```python
from build123d import *

# Parameters (mm, degrees)
SKETCH4_W                       = 152.4
SKETCH4_H                       = 101.6
BOSS_EXTRUDE3_DEPTH             = 6.35
SKETCH5_W                       = 101.6
SKETCH5_H                       = 101.6
BOSS_EXTRUDE4_DEPTH             = 95.25
SKETCH6_W                       = 76.2
SKETCH6_H                       = 76.2
CUT_EXTRUDE1_DEPTH              = 95.25
SKETCH7_R                       = 44.45
BOSS_EXTRUDE5_DEPTH             = 6.35
SKETCH8_R                       = 34.925
CUT_EXTRUDE3_DEPTH              = 171.861025398
CIRPATTERN1_COUNT               = 6
FILLET1_R                       = 3.81
F_4_40_TAPPED_HOLE1_D           = 2.2606
F_4_40_TAPPED_HOLE1_DEPTH       = 8.8646
F_4_40_TAPPED_HOLE1_CSINK_D     = 4.1148
F_4_40_TAPPED_HOLE1_CSINK_ANGLE = 90
F_4_40_TAPPED_HOLE1_TIP         = 0.679152758
SKETCH16_R                      = 19.05
BOSS_EXTRUDE6_DEPTH             = 2.54
CUT_EXTRUDE4_DEPTH              = 175.267880288
CUT_EXTRUDE4_DEPTH_BACK         = 175.267880288
SKETCH17_R                      = 12.7
CUT_EXTRUDE5_DEPTH              = 135.703841816
LPATTERN1_COUNT                 = 2
LPATTERN1_PITCH                 = 76.2


with BuildPart() as part:
    # Sketch4 → Boss-Extrude3 (new body)
    with BuildSketch(Plane(origin=(0, 0, 0), x_dir=(1, 0, 0), z_dir=(0, 1, 0))):
        Rectangle(SKETCH4_W, SKETCH4_H)
    extrude(amount=BOSS_EXTRUDE3_DEPTH)

    # Sketch5 → Boss-Extrude4 (add)
    with BuildSketch(Plane(origin=(0, 6.35, 0), x_dir=(1, 0, 0), z_dir=(0, 1, 0))):
        Rectangle(SKETCH5_W, SKETCH5_H)
    extrude(amount=BOSS_EXTRUDE4_DEPTH)

    # Sketch6 → Cut-Extrude1 (cut)
    with BuildSketch(Plane(origin=(0, 101.6, 0), x_dir=(1, 0, 0), z_dir=(0, 1, 0))):
        Rectangle(SKETCH6_W, SKETCH6_H)
    extrude(amount=-CUT_EXTRUDE1_DEPTH, mode=Mode.SUBTRACT)

    # Sketch7 → Boss-Extrude5 (add)
    with BuildSketch(Plane.XY.offset(50.8)):
        with Locations((0, 50.8)):
            Circle(SKETCH7_R)
    boss_extrude5 = extrude(amount=BOSS_EXTRUDE5_DEPTH)

    # Mirror2: Boss-Extrude5 across plane
    add(boss_extrude5.mirror(Plane.XY))

    # Sketch8 → Cut-Extrude3 (cut, through all)
    with BuildSketch(Plane.XY.offset(57.15)):
        with Locations((0, 50.8)):
            Circle(SKETCH8_R)
    extrude(amount=-CUT_EXTRUDE3_DEPTH, mode=Mode.SUBTRACT)

    # Sketch13 → 1/4-20 Tapped Hole2 (revolve, cut)
    with BuildSketch(Plane(origin=(39.6875, 50.8, 57.15), x_dir=(0, -1, 0), z_dir=(1, 0, 0))):
        Polygon((0, 0), (0, 20.583816902), (2.5527, 19.05), (2.5527, 1.2573), (3.81, 0), align=None)
    f_1_4_20_tapped_hole2 = revolve(axis=Axis((39.6875, 50.8, 63.5), (0, 0, -1)), mode=Mode.SUBTRACT)

    # CirPattern1: 1/4-20 Tapped Hole2 ×6 about axis
    cirpattern1_axis = Axis((0, 50.8, 0), (0, 0, 1))
    for i in range(1, CIRPATTERN1_COUNT):
        add(f_1_4_20_tapped_hole2.rotate(cirpattern1_axis, i * 360 / CIRPATTERN1_COUNT), mode=Mode.SUBTRACT)

    # Fillet1
    fillet1_edges = [part.edges().sort_by_distance(p)[0] for p in [
        (50.8, 53.975, 50.8),
        (50.8, 53.975, -50.8),
        (-50.8, 53.975, -50.8),
        (-50.8, 53.975, 50.8),
    ]]
    fillet(fillet1_edges, radius=FILLET1_R)

    # #4-40 Tapped Hole1
    with Locations(Plane(origin=(0, 101.6, 0), x_dir=(1, 0, 0), z_dir=(0, 1, 0))):
        with Locations((-46.99, 46.99), (46.99, 46.99), (46.99, -46.99), (-46.99, -46.99)):
            CounterSinkHole(F_4_40_TAPPED_HOLE1_D / 2, F_4_40_TAPPED_HOLE1_CSINK_D / 2, depth=F_4_40_TAPPED_HOLE1_DEPTH, counter_sink_angle=F_4_40_TAPPED_HOLE1_CSINK_ANGLE)
            with Locations((0, 0, -(F_4_40_TAPPED_HOLE1_DEPTH + F_4_40_TAPPED_HOLE1_TIP / 2))):  # 118° drill point
                Cone(0, F_4_40_TAPPED_HOLE1_D / 2, F_4_40_TAPPED_HOLE1_TIP, mode=Mode.SUBTRACT)

    # Sketch16 → Boss-Extrude6 (add)
    with BuildSketch(Plane(origin=(50.8, 0, 0), x_dir=(0, 0, -1), z_dir=(1, 0, 0))):
        with Locations(Location((0, 76.2, 0), (0, 0, 180))):
            Circle(SKETCH16_R)
    boss_extrude6 = extrude(amount=BOSS_EXTRUDE6_DEPTH)

    # Mirror4: Boss-Extrude6 across plane
    add(boss_extrude6.mirror(Plane(origin=(0, 0, 0), x_dir=(0, 0, 1), z_dir=(1, 0, 0))))

    # Sketch17 → Cut-Extrude4 (cut, two sides: drawn at the far end of the back side and taken through both)
    with BuildSketch(Plane(origin=(53.34, 0, 0), x_dir=(0, 0, -1), z_dir=(1, 0, 0)).offset(-CUT_EXTRUDE4_DEPTH_BACK)):
        with Locations(Location((0, 76.2, 0), (0, 0, 180))):
            Circle(SKETCH17_R)
    extrude(amount=CUT_EXTRUDE4_DEPTH + CUT_EXTRUDE4_DEPTH_BACK, mode=Mode.SUBTRACT)

    # Mirror5: 1/4-20 Tapped Hole2 across plane
    add(f_1_4_20_tapped_hole2.mirror(Plane.XY), mode=Mode.SUBTRACT)

    # Mirror5 copy 1 sketch → Mirror5 copy 1 (revolve, cut)
    with BuildSketch(Plane(origin=(19.84375, 85.170383213, -57.15), x_dir=(0.8660254037844386, -0.5000000000000001, 0), z_dir=(0.5000000000000001, 0.8660254037844386, 0))):
        Polygon((0, 0), (0, -20.583816902), (2.5527, -19.05), (2.5527, -1.2573), (3.81, 0), align=None)
    revolve(axis=Axis((19.84375, 85.170383213, -63.5), (0, 0, -1)), mode=Mode.SUBTRACT)

    # Mirror5 copy 2 sketch → Mirror5 copy 2 (revolve, cut)
    with BuildSketch(Plane(origin=(-19.84375, 85.170383213, -57.15), x_dir=(0.8660254037844387, 0.4999999999999998, 0), z_dir=(-0.4999999999999998, 0.8660254037844387, 0))):
        Polygon((0, 0), (0, -20.583816902), (2.5527, -19.05), (2.5527, -1.2573), (3.81, 0), align=None)
    revolve(axis=Axis((-19.84375, 85.170383213, -63.5), (0, 0, -1)), mode=Mode.SUBTRACT)

    # Mirror5 copy 3 sketch → Mirror5 copy 3 (revolve, cut)
    with BuildSketch(Plane(origin=(-39.6875, 50.8, -57.15), x_dir=(0, 1, 0), z_dir=(-1, 0, 0))):
        Polygon((0, 0), (0, -20.583816902), (2.5527, -19.05), (2.5527, -1.2573), (3.81, 0), align=None)
    revolve(axis=Axis((-39.6875, 50.8, -63.5), (0, 0, -1)), mode=Mode.SUBTRACT)

    # Mirror5 copy 4 sketch → Mirror5 copy 4 (revolve, cut)
    with BuildSketch(Plane(origin=(-19.84375, 16.429616787, -57.15), x_dir=(-0.8660254037844384, 0.5000000000000004, 0), z_dir=(-0.5000000000000004, -0.8660254037844384, 0))):
        Polygon((0, 0), (0, -20.583816902), (2.5527, -19.05), (2.5527, -1.2573), (3.81, 0), align=None)
    revolve(axis=Axis((-19.84375, 16.429616787, -63.5), (0, 0, -1)), mode=Mode.SUBTRACT)

    # Mirror5 copy 5 sketch → Mirror5 copy 5 (revolve, cut)
    with BuildSketch(Plane(origin=(19.84375, 16.429616787, -57.15), x_dir=(-0.8660254037844386, -0.5000000000000001, 0), z_dir=(0.5000000000000001, -0.8660254037844386, 0))):
        Polygon((0, 0), (0, -20.583816902), (2.5527, -19.05), (2.5527, -1.2573), (3.81, 0), align=None)
    revolve(axis=Axis((19.84375, 16.429616787, -63.5), (0, 0, -1)), mode=Mode.SUBTRACT)

    # Sketch19 → Cut-Extrude5 (cut, through all)
    with BuildSketch(Plane(origin=(0, 6.35, 0), x_dir=(1, 0, 0), z_dir=(0, 1, 0))):
        with BuildLine():
            Line((69.85, -30.48), (69.85, -43.18))
            ThreePointArc((69.85, -43.18), (66.675, -46.355), (63.5, -43.18))
            Line((63.5, -43.18), (63.5, -30.48))
            ThreePointArc((63.5, -30.48), (66.675, -27.305), (69.85, -30.48))
        make_face()
    cut_extrude5 = extrude(amount=-CUT_EXTRUDE5_DEPTH, mode=Mode.SUBTRACT)

    # LPattern1: Cut-Extrude5 ×2
    with Locations(*[(0, 0, -i * LPATTERN1_PITCH) for i in range(1, LPATTERN1_COUNT)]):
        add(cut_extrude5, mode=Mode.SUBTRACT)


solid = part.part
```
The listing builds one solid part. Answer for the finished solid, in the listing's coordinates (mm). A direction names the side the tool comes from. Coordinates: 2 decimals unless noted, no trailing zeros. Write each loop counter-clockwise with the first axis right and the second up, starting at its lowest first coordinate (ties: lowest second). Pieces come first, ordered by that corner, then holes. Notation, with made-up numbers: (79.25, 52.25) - (134.25, 52.25) arc R18 cw to (134.25, 59.25) - close; hole circle Ø5 at (69, 86.25). An arc over 180 degrees is marked (long way). Return JSON: item names as keys, results as strings. Group by question number.
Q1. Find the intervals of material crossed by line 1 along X through (y, z) = (37, -4); line 2 along Z through (x, y) = (-3.5, 7), in increasing order. Write a range as [from, to].
Q2. For a pull along Z with two mould halves and no side action, classify faces 6 (the cylindrical face through (66.745, 3.219, -29.846)), 7 (the cylindrical face through (-49.654, 54.642, 49.714)), 8 (the cylindrical face through (-49.654, 54.642, -49.714)), 9 (the flat face through (-50.8, 53, 1)) as +Z half, -Z half, draft (parallel to the pull), parting line (faces both ways), or undercut.
Q3. The part is cut by section A-A on x = 0. Write down the section's boundary in (y, z) (3 decimals), and give its area (3 significant figures).
Q4. The part is cut by section C-C on y = 39.5. Write down the section's boundary in (x, z), and give its area (3 significant figures).
Q5. The part is cut by section B-B on z = 0. Write down the section's boundary in (x, y), and give its area (3 significant figures).
Q6. Flat-ended cylindrical pins translate along their axes: pin 1 Ø23 at (y, z) = (76.2, 0) entering from +X; pin 2 Ø1 at (x, z) = (-60, -43.5) entering from +Y; pin 3 Ø3 at (x, z) = (46.99, 46.99) entering from +Y; pin 4 Ø12 at (x, y) = (-47, 86) entering from -Z. Find the tip coordinate at first contact, or state that the pin passes through.
Q7. Which of the six approach directions +Z, -Z, +X, -X, +Y, -Y give full straight-line access (tool end or side, diameter ignored) to faces 1 (the cylindrical face through (-9.6, 7.4, 53.9)), 2 (the cylindrical face through (49.654, 54.642, -49.714)), 3 (the flat face through (38.1, 55, 1)), 4 (the cylindrical face through (66.605, 3.219, -48.894)), 5 (the cylindrical face through (-42.18, 50.25, -47.12))?
Q8. The part is cut by section D-D on x = 25.5. Write down the section's boundary in (y, z).
Evaluation:
{
 "1": {"line 1": "x = [-50.8, -38.1], [38.1, 50.8]", "line 2": "z = [-57.15, -38.1], [38.1, 57.15]"},
 "2": {"face 6": "undercut", "face 7": "+Z half", "face 8": "-Z half", "face 9": "draft"},
 "3": {"outline": "(0, -50.8) - (6.35, -50.8) - (6.35, -57.15) - (15.875, -57.15) - (15.875, -38.1) - (6.35, -38.1) - (6.35, 38.1) - (15.875, 38.1) - (15.875, 57.15) - (6.35, 57.15) - (6.35, 50.8) - (0, 50.8) - close; (85.725, -57.15) - (95.25, -57.15) - (95.25, -50.8) - (101.6, -50.8) - (101.6, -38.1) - (85.725, -38.1) - close; (85.725, 38.1) - (101.6, 38.1) - (101.6, 50.8) - (95.25, 50.8) - (95.25, 57.15) - (85.725, 57.15) - close", "area": "1,530 mm2"},
 "4": {"outline": "(-50.8, -46.99) arc R3.81 ccw to (-46.99, -50.8) - (-42.99, -50.8) - (-42.99, -57.15) - (-33.05, -57.15) - (-33.05, -38.1) - (-38.1, -38.1) - (-38.1, 38.1) - (-33.05, 38.1) - (-33.05, 57.15) - (-42.99, 57.15) - (-42.99, 50.8) - (-46.99, 50.8) arc R3.81 ccw to (-50.8, 46.99) - close; (33.05, -57.15) - (42.99, -57.15) - (42.99, -50.8) - (46.99, -50.8) arc R3.81 ccw to (50.8, -46.99) - (50.8, 46.99) arc R3.81 ccw to (46.99, 50.8) - (42.99, 50.8) - (42.99, 57.15) - (33.05, 57.15) - (33.05, 38.1) - (38.1, 38.1) - (38.1, -38.1) - (33.05, -38.1) - close", "area": "3,080 mm2"},
 "5": {"outline": "(-76.2, 0) - (76.2, 0) - (76.2, 6.35) - (50.8, 6.35) - (50.8, 57.15) - (53.34, 57.15) - (53.34, 63.5) - (38.1, 63.5) - (38.1, 6.35) - (-38.1, 6.35) - (-38.1, 63.5) - (-53.34, 63.5) - (-53.34, 57.15) - (-50.8, 57.15) - (-50.8, 6.35) - (-76.2, 6.35) - close; (-53.34, 88.9) - (-38.1, 88.9) - (-38.1, 101.6) - (-50.8, 101.6) - (-50.8, 95.25) - (-53.34, 95.25) - close; (38.1, 88.9) - (53.34, 88.9) - (53.34, 95.25) - (50.8, 95.25) - (50.8, 101.6) - (38.1, 101.6) - close", "area": "2,810 mm2"},
 "6": {"pin 1": "passes through", "pin 2": "stops at y = 6.35", "pin 3": "stops at y = 101.04", "pin 4": "stops at z = -50.8"},
 "7": {"face 1": "+Z", "face 2": "-Z, +X, +Y", "face 3": "+Y", "face 4": "+Y, -Y", "face 5": "-Z"},
 "8": {"outline": "(0, -50.8) - (14.39, -50.8) - (14.39, -57.15) - (26.94, -57.15) - (26.94, -38.1) - (6.35, -38.1) - (6.35, 38.1) - (26.94, 38.1) - (26.94, 57.15) - (14.39, 57.15) - (14.39, 50.8) - (0, 50.8) - close; (74.66, -57.15) - (87.21, -57.15) - (87.21, -50.8) - (101.6, -50.8) - (101.6, -38.1) - (74.66, -38.1) - close; (74.66, 38.1) - (101.6, 38.1) - (101.6, 50.8) - (87.21, 50.8) - (87.21, 57.15) - (74.66, 57.15) - close"}
}
